Here's how the part is built. I have some questions about the finished solid (model axes, mm). A direction names the side the tool comes from. Give positions to 0.01 mm unless a question says otherwise; leave off trailing zeros. Write each loop counter-clockwise with the first axis right and the second up, starting at its lowest first coordinate (ties: lowest second). Pieces come first, ordered by that corner, then holes. Notation, with made-up numbers: (-38, 15.25) -> (5, 15.25) arc R28 ccw to (5, 53.25) -> close; hole circle Ø3 at (-22.75, 24). An arc over 180 degrees is marked (long way). Use one line per item in the form item = value.
```python
from build123d import *

# Parameters (mm, degrees)
SKETCH_1_R           = 18.5
SKETCH_1_R_2         = 13.5
EXTRUDE_1_DEPTH      = 10
EXTRUDE_2_REACH      = 50.317
EXTRUDE_2_END_RADIUS = 18.5
SKETCH_2_R           = 7.5
SKETCH_3_W           = 30
SKETCH_3_H           = 30
EXTRUDE_3_DEPTH      = 10
SKETCH_4_R           = 2
CUT_EXTRUDE_1_DEPTH  = 15
SKETCH_5_R           = 4.5
CUT_EXTRUDE_2_DEPTH  = 1.5


with BuildPart() as part:
    # 草图1 → 凸台-拉伸1 (new, symmetric)
    with BuildSketch(Plane.XY):
        Circle(SKETCH_1_R)
        Circle(SKETCH_1_R_2, mode=Mode.SUBTRACT)
    extrude(amount=EXTRUDE_1_DEPTH, both=True)

    # 凸台-拉伸2: up to this cylinder (the profile starts outside it)
    extrude_2_end = Plane(origin=(0, 0, 0), z_dir=(0, 0, -1)) * Cylinder(EXTRUDE_2_END_RADIUS, 138.634, mode=Mode.PRIVATE)
    # 草图2 → 凸台-拉伸2 (add, up to the surface)
    with BuildSketch(Plane(origin=(0, -25, 0), x_dir=(1, 0, 0), z_dir=(0, 1, 0)), mode=Mode.PRIVATE) as extrude_2_sk1:
        with Locations(Location((0, 0, 0), (0, 0, 90))):
            Circle(SKETCH_2_R)
    extrude_2_tool1 = extrude(extrude_2_sk1.sketch, amount=EXTRUDE_2_REACH, mode=Mode.PRIVATE) - extrude_2_end
    add(extrude_2_tool1.solids().sort_by_distance((0, -25, 0))[0])

    # 草图3 → 凸台-拉伸3 (add)
    with BuildSketch(Plane.XZ.offset(25)):
        Rectangle(SKETCH_3_W, SKETCH_3_H)
    extrude(amount=EXTRUDE_3_DEPTH)

    # 草图4 → 切除-拉伸1 (cut)
    with BuildSketch(Plane.XZ.offset(35)):
        with Locations(Location((-9.270440252, 10, 0), (0, 0, 270))):
            Circle(SKETCH_4_R)
        with Locations(Location((9.270440252, 10, 0), (0, 0, 270))):
            Circle(SKETCH_4_R)
        with Locations(Location((-9.270440252, -10, 0), (0, 0, 270))):
            Circle(SKETCH_4_R)
        with Locations(Location((9.270440252, -10, 0), (0, 0, 270))):
            Circle(SKETCH_4_R)
    extrude(amount=-CUT_EXTRUDE_1_DEPTH, mode=Mode.SUBTRACT)

    # 草图5 → 切除-拉伸2 (cut)
    with BuildSketch(Plane(origin=(0, -25, 0), x_dir=(1, 0, 0), z_dir=(0, 1, 0))):
        with Locations(Location((-9.270440252, -10, 0), (0, 0, 270))):
            Circle(SKETCH_5_R)
        with Locations(Location((9.270440252, -10, 0), (0, 0, 270))):
            Circle(SKETCH_5_R)
        with Locations(Location((9.270440252, 10, 0), (0, 0, 270))):
            Circle(SKETCH_5_R)
        with Locations(Location((-9.270440252, 10, 0), (0, 0, 270))):
            Circle(SKETCH_5_R)
    extrude(amount=-CUT_EXTRUDE_2_DEPTH, mode=Mode.SUBTRACT)


solid = part.part
```
Q1. Which directions (+Z, -Z, +X, -X, +Y, -Y) give clear straight access to the entire face, cutting with the end or side of a thin tool? Please do faces 4 (the face through (15, -30, 0)), 5 (the face through (-7.287, -30.81, -9.74)), 6 (the face through (2.87, -21.01, -6.93)), 7 (the face through (-15, -30, 0)).
Result set:
face_4 = +Z, -Z, +X, -Y
face_5 = -Y
face_6 = none
face_7 = +Z, -Z, -X, -Y
Q2. If we mould it in two halves opening along Z, with no side actions, what happens to faces 1 (the face through (1, -14, -10)), 2 (the face through (8, -26.5, -8)), 3 (the face through (1, -14, 10))? For each: +Z half, -Z half, draft (parallel to the pull), parting line (faces both ways), or undercut.
Result set:
face_1 = -Z half
face_2 = undercut
face_3 = +Z half
Q3. I want a section at A-A, the plane x = 0. Write out the boundary of the cut face in (y, z).
Result set:
outline = (-35, -15) -> (-25, -15) -> (-25, -7.5) -> (-18.5, -7.5) -> (-18.5, -10) -> (-13.5, -10) -> (-13.5, 10) -> (-18.5, 10) -> (-18.5, 7.5) -> (-25, 7.5) -> (-25, 15) -> (-35, 15) -> close; (13.5, -10) -> (18.5, -10) -> (18.5, 10) -> (13.5, 10) -> close
Q4. I want a section at B-B, the plane z = 0. Write out the boundary of the cut face in (x, y).
Result set:
outline = (-15, -35) -> (15, -35) -> (15, -25) -> (7.5, -25) -> (7.5, -16.91) arc R18.5 ccw (long way) to (-7.5, -16.91) -> (-7.5, -25) -> (-15, -25) -> close; hole circle Ø27 at (0, 0)
Q5. I want a section at D-D, the plane z = 9. Write out the boundary of the cut face in (x, y), and give its area (3 significant figures).
Result set:
outline = circle Ø37 at (0, 0); (-15, -35) -> (-11, -35) -> (-11, -26.5) -> (-13.66, -26.5) -> (-13.66, -25) -> (-15, -25) -> close; (-7.54, -35) -> (7.54, -35) -> (7.54, -26.5) -> (4.88, -26.5) -> (4.88, -25) -> (-4.88, -25) -> (-4.88, -26.5) -> (-7.54, -26.5) -> close; (11, -35) -> (15, -35) -> (15, -25) -> (13.66, -25) -> (13.66, -26.5) -> (11, -26.5) -> close; hole circle Ø27 at (0, 0)
area = 717 mm2
Q6. If I drill on line 1 along X through (y, z) = (-26, -10); line 2 along X through (y, z) = (-29, 10); line 3 along X through (y, z) = (0.5, -9.5), over which ranges is the centre line in solid material (lowest first)? Write a range as from..to.
Result set:
line_1 = -15..-13.77, -4.77..4.77, 13.77..15
line_2 = -15..-11.27, -7.27..7.27, 11.27..15
line_3 = -18.49..-13.49, 13.49..18.49
Q7. Will these pins go through, and if not, where does the flat tip stop? pin 1 Ø3.5 at (x, z) = (9.27, -10) entering from -Y; pin 2 Ø1.5 at (y, z) = (11, -8.5) entering from +X; pin 3 Ø7 at (x, z) = (-10.5, -10) entering from +Y.
Result set:
pin_1 = -16.9
pin_2 = 15.4
pin_3 = 17.12
Q8. I want a section at C-C, the plane y = 0. Write out the boundary of the cut face in (x, z).
Result set:
outline = (-18.5, -10) -> (-13.5, -10) -> (-13.5, 10) -> (-18.5, 10) -> close; (13.5, -10) -> (18.5, -10) -> (18.5, 10) -> (13.5, 10) -> close
